The listing builds one solid part. Answer for the finished solid, in the listing's coordinates (mm). A direction names the side the tool comes from. Coordinates: 2 decimals unless noted, no trailing zeros. Write each loop counter-clockwise with the first axis right and the second up, starting at its lowest first coordinate (ties: lowest second). Pieces come first, ordered by that corner, then holes.
```python
from build123d import *

# Parameters (mm, degrees)
BOSS_EXTRUDE1_DEPTH                     = 4
CBORE_FOR_M5_HEX_HEAD_BOLT1_D           = 2.7
CBORE_FOR_M5_HEX_HEAD_BOLT1_CBORE_D     = 5
CBORE_FOR_M5_HEX_HEAD_BOLT1_CBORE_DEPTH = 2
SKETCH6_R                               = 1.75
BOSS_EXTRUDE2_DEPTH                     = 4
FILLET1_R                               = 5.5
FILLET1_OF_MIRROR1_R                    = 5.5
FILLET2_R                               = 1.8
FILLET3_R                               = 1


with BuildPart() as part:
    # Sketch2 → Boss-Extrude1 (new body)
    with BuildSketch(Plane.XY):
        with BuildLine():
            Line((-18.3, -1.2), (18.3, -1.2))
            Line((18.3, -1.2), (18.3, 43.8))
            add(Edge.make_bspline(
                [(18.3, 43.8), (18.3, 58.8), (6.363961031, 74.436038969), (0, 80.8)],
                knots=[0, 0, 0, 0, 1, 1, 1, 1], degree=3))
            add(Edge.make_bspline(
                [(-18.3, 43.8), (-18.3, 58.8), (-6.363961031, 74.436038969), (0, 80.8)],
                knots=[0, 0, 0, 0, 1, 1, 1, 1], degree=3))
            Line((-18.3, 43.8), (-18.3, -1.2))
        make_face()
    extrude(amount=BOSS_EXTRUDE1_DEPTH)

    # CBORE for M5 Hex Head Bolt1 (through all)
    with Locations(Plane(origin=(0, 0, 0), x_dir=(-1, 0, 0), z_dir=(0, 0, -1))):
        with Locations((14.4, 42.017834424), (14.4, 2.863521172), (-14.4, 2.863521172), (-14.4, 42.017834424), (0, 74.6)):
            CounterBoreHole(CBORE_FOR_M5_HEX_HEAD_BOLT1_D / 2, CBORE_FOR_M5_HEX_HEAD_BOLT1_CBORE_D / 2, CBORE_FOR_M5_HEX_HEAD_BOLT1_CBORE_DEPTH)

    # Sketch6 → Boss-Extrude2 (add)
    with BuildSketch(Plane(origin=(7, 0, 0), x_dir=(0, 0, -1), z_dir=(1, 0, 0))):
        with BuildLine():
            Line((0, 44.8), (5.5, 44.8))
            ThreePointArc((5.5, 44.8), (10.5, 39.8), (5.5, 34.8))
            Line((5.5, 34.8), (0, 34.8))
            Line((0, 34.8), (0, 44.8))
        make_face()
        with Locations((5.5, 39.8)):
            Circle(SKETCH6_R, mode=Mode.SUBTRACT)
    boss_extrude2 = extrude(amount=-BOSS_EXTRUDE2_DEPTH)

    # Fillet1
    fillet1_edges = [part.edges().sort_by_distance(p)[0] for p in [
        (5, 34.8, 0),
        (5, 44.8, 0),
    ]]
    fillet(fillet1_edges, radius=FILLET1_R - 0.0001)  # a hair under: the kernel refuses the full size

    # Mirror1: Boss-Extrude2 across plane
    add(boss_extrude2.mirror(Plane(origin=(0, 0, 0), x_dir=(0, 0, 1), z_dir=(1, 0, 0))))

    # Fillet1 of Mirror1
    fillet1_of_mirror1_edges = [part.edges().sort_by_distance(p)[0] for p in [
        (-5, 34.8, 0),
        (-5, 44.8, 0),
    ]]
    fillet(fillet1_of_mirror1_edges, radius=FILLET1_OF_MIRROR1_R - 0.0001)  # a hair under: the kernel refuses the full size

    # Fillet2
    fillet2_edges = [part.edges().sort_by_distance(p)[0] for p in [
        (0, 80.8, 2),
    ]]
    fillet(fillet2_edges, radius=FILLET2_R)

    # Fillet3
    fillet3_edges = [part.edges().sort_by_distance(p)[0] for p in [
        (18.3, -1.2, 2),
        (-18.3, -1.2, 2),
    ]]
    fillet(fillet3_edges, radius=FILLET3_R)


solid = part.part
```
(1) Which of the six approach directions +Z, -Z, +X, -X, +Y, -Y give full straight-line access (tool end or side, diameter ignored) to faces 1 (the flat face through (18.3, 21, 2)), 2 (the flat face through (13, 2, 2)), 3 (the flat face through (7, 40, -3))?
(2) Section D-D, the plane z = -1.75 is taken. Write down the section's boundary in (x, y).
(3) Section B-B, the plane x = 14.4 is taken. State how many separate pieces and enclosed holes the cut face has, plus the area to 3 significant figures.
(4) Find the intervals of material crossed by probe 1 along Y at (x, z) = (0, 0.95); probe 2 along X at (y, z) = (45, -3.5); probe 3 along Z at (x, y) = (0, 60.5), in increasing order.
(5) Section C-C, the plane y = 18 is taken. Write down the section's boundary in (x, z).
(6) Section A-A, the plane z = -8 is taken. Write down the section's boundary in (x, y), plus the area to 3 significant figures.
(7) Each of these flat-tipped pins is pushed along its axis until it touches: pin 1 (5.5 mm diameter, centred on x = -15, y = 3, fed in from -Z); pin 2 (4 mm diameter, centred on y = 47.5, z = 0, fed in from +X); pin 3 (4.5 mm diameter, centred on x = -14.4, y = 2.86, fed in from -Z). Where does it stop, or does it pass through?
(8) For a pull along Y with two mould halves and no side action, classify faces 4 (the cylindrical face through (-4.97, 33.15, -1.57)), 5 (the cylindrical face through (-14.693, 1.546, 3.014)), 6 (the flat face through (0, 31, 0)) as pulls with the +Y half, pulls with the -Y half, needs draft (parallel to the pull), parting line crosses it, or undercut.
Solution:
1. face 1: +Z, -Z, +X, +Y, -Y
1. face 2: -Z
1. face 3: -Z, +X, +Y, -Y
2. outline: (-7, 33.32) - (-3, 33.32) - (-3, 46.28) - (-7, 46.28) - close; (3, 33.32) - (7, 33.32) - (7, 46.28) - (3, 46.28) - close
3. separate pieces: 3
3. enclosed holes: 0
3. area: 214 mm2
4. probe 1: y = -1.2 to 72.1, 77.1 to 80.01
4. probe 2: x = -7 to -3, 3 to 7
4. probe 3: z = 0 to 4
5. outline: (-18.3, 0) - (18.3, 0) - (18.3, 4) - (-18.3, 4) - close
6. outline: (-7, 35.47) - (-3, 35.47) - (-3, 44.13) - (-7, 44.13) - close; (3, 35.47) - (7, 35.47) - (7, 44.13) - (3, 44.13) - close
6. area: 69.3 mm2
7. pin 1: stops at z = 0
7. pin 2: stops at x = 18.25
7. pin 3: stops at z = 2
8. face 4: pulls with the -Y half
8. face 5: undercut
8. face 6: needs draft
